Geometry check sheet. Reference: the model listing, model coordinates, mm. A direction names the side the tool comes from. Round coordinates to 2 decimals unless told otherwise and drop trailing zeros. Order: outer loops, then holes, each group sorted by start corner. A loop starts at its lowest first (then second) coordinate and runs counter-clockwise, first axis right, second up. Notation, with made-up numbers: (7.5, 61.5) -> (31.5, 61.5) arc R8 cw to (31.5, 70.5) -> close; hole circle Ø8 at (3, 63.5). An arc over 180 degrees is marked (long way). Use a Markdown table: item, result. Add a question column.
Item 1: Sectioned sample at A-A, the plane y = 2.3. State how many separate pieces and enclosed holes the cut face has, and give its area (3 significant figures).
Item 2: Set-up check for faces 1 (the flat face through (-43.75, 1, -139)), 2 (the flat face through (-3, 1, -26)), 3 (the flat face through (-1, 1, -122.5)): record each of +Z, -Z, +X, -X, +Y, -Y from which the full face is reachable in a straight line by a thin tool's end or side.
Item 3: Sectioned sample at C-C, the plane x = -72. Record the cut outline in (y, z), and give its area (3 significant figures).
Item 4: Material ranges on probe 1 along X at (y, z) = (1.35, -104); probe 2 along Z at (x, y) = (-77.75, 1.4); probe 3 along X at (y, z) = (1.3, -36), recorded low to high. Write a range as [from, to].
Item 5: Mould release check, pull along Z, two halves, no side actions. Record for faces 4 (the flat face through (-105, 1, -114)), 5 (the flat face through (-6, 1, -137)), 6 (the flat face through (-102, 1, -26)): pulls with the +Z half, pulls with the -Z half, needs draft (parallel to the pull), parting line crosses it, or undercut.
Item 6: Sectioned sample at B-B, the plane z = -28. Record the cut outline in (x, y), and give its area (3 significant figures).
Item 7: Gauge pin test, flat ends, axial feed: pin 1 Ø0.9 at (x, y) = (-1, 1.5) entering from +Z; pin 2 Ø1.5 at (y, z) = (2, -123.5) entering from +X; pin 3 Ø1.5 at (x, y) = (-104, 2) entering from -Z; pin 4 Ø1.5 at (x, y) = (-7, 1.5) entering from -Z. Record the tip position at first contact, or that the pin passes through.
Autodesk Inventor part; units mm, degrees
ref_plane "YZ Plane" through (0, 0, 0) normal (1, 0, 0) x (0, 1, 0)
ref_plane "XZ Plane" through (0, 0, 0) normal (0, 1, 0) x (-1, 0, 0)
ref_plane "XY Plane" through (0, 0, 0) normal (0, 0, 1) x (1, 0, 0)
sketch "Sketch2" plane through (0, 0, 0) normal (0, 1, 0) x (-1, 0, 0)
  line L0 (0, 0) -> (105, 0)
  line L1 (105, 0) -> (105, -140)
  line L2 (105, -140) -> (0, -140)
  line L3 (0, -140) -> (0, 0)
  point P0 (75, -100)
  dimension "d4" = 105
  dimension "d5" = 140
extrude "Extrusion2" add sketch "Sketch2" along normal blind 3
sketch "Sketch3" plane through (0, 0, 0) normal (0, -1, 0) x (1, 0, 0)
  line L0 (-105, 0) -> (0, 0)
  line L1 (-105, -140) -> (-105, 0)
  line L2 (0, -17.5) -> (-3, -17.5)
  line L3 (-3, -17.5) -> (-3, -35)
  line L4 (-3, -35) -> (0, -35)
  line L5 (0, -35) -> (0, -52.5)
  line L6 (0, -52.5) -> (-3, -52.5)
  line L7 (-3, -52.5) -> (-3, -70)
  line L8 (-3, -70) -> (0, -70)
  line L9 (0, -70) -> (0, -87.5)
  line L10 (0, -87.5) -> (-3, -87.5)
  line L11 (-3, -87.5) -> (-3, -105)
  line L12 (-3, -105) -> (0, -105)
  line L13 (0, -105) -> (0, -122.5)
  line L14 (0, -122.5) -> (-3, -122.5)
  line L15 (-3, -122.5) -> (-3, -140)
  line L16 (0, -17.5) -> (0, 0)
  line L17 (-105, 0) -> (0, 0)
  line L18 (-105, -140) -> (-105, 0)
  line L19 (0, 0) -> (-105, 0)
  line L20 (-105, 0) -> (-105, -17.5)
  line L21 (-105, -17.5) -> (-102, -17.5)
  line L22 (-102, -17.5) -> (-102, -35)
  line L23 (-102, -35) -> (-105, -35)
  line L24 (-105, -35) -> (-105, -52.5)
  line L25 (-102, -52.5) -> (-105, -52.5)
  line L26 (-102, -52.5) -> (-102, -70)
  line L27 (-102, -70) -> (-105, -70)
  line L28 (-105, -70) -> (-105, -87.5)
  line L29 (-105, -87.5) -> (-102, -87.5)
  line L30 (-102, -87.5) -> (-102, -105)
  line L31 (-102, -105) -> (-105, -105)
  line L32 (-105, -105) -> (-105, -122.5)
  line L33 (-105, -122.5) -> (-102, -122.5)
  line L34 (-102, -122.5) -> (-102, -137)
  line L35 (0, -140) -> (-105, -140)
  line L36 (-105, -122.5) -> (-105, -105)
  line L37 (-102, -137) -> (-96.25, -137)
  line L38 (-96.25, -137) -> (-96.25, -140)
  line L39 (-96.25, -140) -> (-78.75, -140)
  line L40 (-52.5, -140) -> (-35, -140)
  line L41 (-17.5, -140) -> (-3, -140)
  line L42 (-3, -140) -> (-3, -137)
  line L43 (-61.25, -140) -> (-43.75, -140)
  line L44 (-43.75, -140) -> (-43.75, -137)
  line L45 (-43.75, -137) -> (-26.25, -137)
  line L46 (-26.25, -137) -> (-26.25, -140)
  line L47 (-26.25, -140) -> (-8.75, -140)
  line L48 (-8.75, -140) -> (-8.75, -137)
  line L49 (-8.75, -137) -> (-3, -137)
  line L50 (-96.25, -137) -> (-96.25, -140)
  line L51 (-96.25, -140) -> (-78.75, -140)
  line L52 (-78.75, -140) -> (-78.75, -137)
  line L53 (-78.75, -137) -> (-61.25, -137)
  line L54 (-61.25, -137) -> (-61.25, -140)
  line L55 (-61.25, -140) -> (-43.75, -140)
  line L56 (-26.25, -140) -> (-8.75, -140)
  point P0 (-17.5, -137)
  dimension "d51" = 3
  dimension "d52" = 17.5
  dimension "d53" = 17.5
  dimension "d54" = 17.5
  dimension "d55" = 17.5
  dimension "d56" = 17.5
  dimension "d58" = 3
  dimension "d65" = 17.5
  dimension "d66" = 17.5
  dimension "d67" = 17.5
  dimension "d69" = 5.75
  dimension "d70" = 5.75
  dimension "d71" = 17.5
extrude "Extrusion3" cut sketch "Sketch3" against normal blind 3 contours L0 L16 L2 L3 L4 L5 L6 L7 L8 L9 L10 L11 L12 L13 L14 L15 L49 L48 L35 L46 L45 L44 L54 L53 L52 L38 L37 L34 L33 L1 L31 L30 L29 L27 L26 L25 L23 L22 L21 keep common part
sketch "Sketch5" plane through (0, 3, 0) normal (0, 1, 0) x (1, 0, 0)
  circle A0 centre (-27.25, 36) radius 3
  line L0 (0, 0) -> (0, 17.5)
  line L1 (0, 0) -> (0, 17.5)
  line L2 (-105, 0) -> (0, 0)
  line L3 (0, 0) -> (-17.5, 0)
  circle A1 centre (-77.75, 36) radius 3
  circle A2 centre (-27.25, 104) radius 3
  circle A3 centre (-77.75, 104) radius 3
  line L4 (-3, 122.5) -> (-3, 137)
  line L5 (-26.25, 137) -> (-43.75, 137)
  line L6 (0, 105) -> (0, 122.5)
  line L7 (-8.75, 140) -> (-26.25, 140)
  dimension "d72" = 17.5
  dimension "d75" = 50.5
  dimension "d78" = 68
  dimension "d81" = 6
  dimension "d84" = 27.25
  dimension "d85" = 36
extrude "Extrusion4" cut sketch "Sketch5" against normal blind 2.5
properties part number "TableBottom" material "Wood (Cherry)"
Found:
| question | item | result |
|---|---|---|
| 1 | separate pieces | 1 |
| 1 | enclosed holes | 4 |
| 1 | area | 14,000 mm2 |
| 2 | face 1 | -Z, +Y, -Y |
| 2 | face 2 | +X, +Y, -Y |
| 2 | face 3 | -Z, +X, +Y, -Y |
| 3 | outline | (0, -137) -> (3, -137) -> (3, 0) -> (0, 0) -> close |
| 3 | area | 411 mm2 |
| 4 | probe 1 | x = [-102, -80.75], [-74.75, -30.25], [-24.25, -3] |
| 4 | probe 2 | z = [-137, -107], [-101, -39], [-33, 0] |
| 4 | probe 3 | x = [-105, -80.75], [-74.75, -30.25], [-24.25, 0] |
| 5 | face 4 | needs draft |
| 5 | face 5 | pulls with the -Z half |
| 5 | face 6 | undercut |
| 6 | outline | (-102, 0) -> (-3, 0) -> (-3, 3) -> (-102, 3) -> close |
| 6 | area | 297 mm2 |
| 7 | pin 1 | stops at z = 0 |
| 7 | pin 2 | stops at x = -3 |
| 7 | pin 3 | stops at z = -122.5 |
| 7 | pin 4 | stops at z = -137 |
